from build123d import *

# Parameters (mm, degrees)
SKETCH_W        = 60
SKETCH_H        = 60
PAD_DEPTH       = 4
SKETCH001_W     = 60
SKETCH001_H     = 60
SKETCH001_W_2   = 51
SKETCH001_H_2   = 51
PAD001_DEPTH    = 16
SKETCH002_R     = 15
POCKET_DEPTH    = 5
SKETCH003_R     = 2.5
POCKET001_DEPTH = 5


with BuildPart() as part:
    # Sketch → Pad (new body)
    with BuildSketch(Plane.XY):
        with Locations((20, -20)):
            Rectangle(SKETCH_W, SKETCH_H)
    extrude(amount=PAD_DEPTH)

    # Sketch001 (on Face6 of Pad) → Pad001 (join)
    with BuildSketch(Plane.XY.offset(4)):
        with Locations((20, -20)):
            Rectangle(SKETCH001_W, SKETCH001_H)
        with Locations((19.5, -19.5)):
            Rectangle(SKETCH001_W_2, SKETCH001_H_2, mode=Mode.SUBTRACT)
    extrude(amount=PAD001_DEPTH)

    # Sketch002 (on Face4 of Pad001) → Pocket (cut)
    with BuildSketch(Plane(origin=(0, 0, 0), x_dir=(1, 0, 0), z_dir=(0, 0, -1))):
        with Locations((25, 25)):
            Circle(SKETCH002_R)
    extrude(amount=-POCKET_DEPTH, mode=Mode.SUBTRACT)

    # Sketch003 (on Face4 of Pocket) → Pocket001 (cut)
    with BuildSketch(Plane(origin=(0, 0, 0), x_dir=(1, 0, 0), z_dir=(0, 0, -1))):
        with Locations((7.960481, 8.281351)):
            Circle(SKETCH003_R)
    extrude(amount=-POCKET001_DEPTH, mode=Mode.SUBTRACT)


solid = part.part
Source: CAD feature listing. Evaluate the final solid. Frame: model axes, mm. A direction names the side the tool comes from. Round coordinates to 2 decimals unless told otherwise and drop trailing zeros. Order: outer loops, then holes, each group sorted by start corner. A loop starts at its lowest first (then second) coordinate and runs counter-clockwise, first axis right, second up. Notation, with made-up numbers: (62, 45) - (115, 45) arc R26 cw to (115, 61) - close; hole circle Ø3 at (48, -2.75). An arc over 180 degrees is marked (long way). Use a Markdown table: item, result. Add a question column.
1. First-contact query: pin 1 (1.5 mm diameter, centred on x = 10.5, y = -36.5, fed in from +Z). Flat tip, straight axial feed; report the tip coordinate or a pass-through.
2. Set-up query: faces 1 (the flat face through (19, 6, 12)), 2 (the flat face through (-10, -20, 10)). Return all of +Z, -Z, +X, -X, +Y, -Y with unobstructed straight access to the full face (end or side cutting, diameter ignored); none if empty.
3. Section query A-A (x = 25). Return the cut outline in (y, z).
4. Section query D-D (x = -5). Return the cut outline in (y, z).
5. Section query B-B (y = -25). Return the cut outline in (x, z), then the cut area to 3 significant figures.
6. Line query: probe 1 along Y at (x, z) = (43, 7.75); probe 2 along X at (y, z) = (-43, 9); probe 3 along Y at (x, z) = (25, 2.45). Output: solid intervals per line, ascending.
7. Section query C-C (z = 16). Return the cut outline in (x, y).
Derived:
| question | item | result |
|---|---|---|
| 1 | pin 1 | z = 4 |
| 2 | face 1 | +Z |
| 2 | face 2 | +Z, -Z, -X, +Y, -Y |
| 3 | outline | (-50, 0) - (-40, 0) - (-40, 4) - (-45, 4) - (-45, 20) - (-50, 20) - close; (-10, 0) - (10, 0) - (10, 20) - (6, 20) - (6, 4) - (-10, 4) - close |
| 4 | outline | (-50, 0) - (10, 0) - (10, 20) - (6, 20) - (6, 4) - (-45, 4) - (-45, 20) - (-50, 20) - close |
| 5 | outline | (-10, 0) - (10, 0) - (10, 4) - (-6, 4) - (-6, 20) - (-10, 20) - close; (40, 0) - (50, 0) - (50, 20) - (45, 20) - (45, 4) - (40, 4) - close |
| 5 | area | 264 mm2 |
| 6 | probe 1 | -50 to -45, 6 to 10 |
| 6 | probe 2 | -10 to -6, 45 to 50 |
| 6 | probe 3 | -50 to -40, -10 to 10 |
| 7 | outline | (-10, -50) - (50, -50) - (50, 10) - (-10, 10) - close; hole (-6, -45) - (45, -45) - (45, 6) - (-6, 6) - close |
